Answer from the drawing. Dimensions are ordinates in mm from the lowest x, y and z of the part. A direction names the side the tool comes from. Give positions to 0.01 mm unless a question says otherwise; leave off trailing zeros. Order: outer loops, then holes, each group sorted by start corner. A loop starts at its lowest first (then second) coordinate and runs counter-clockwise, first axis right, second up. Notation, with made-up numbers: (-25, 25.25) - (34, 25.25) arc R32 ccw to (34, 62.25) - close; hole circle Ø2 at (49.25, 24.5). An arc over 180 degrees is marked (long way). One line per item, written item: value. Start each with the question number.
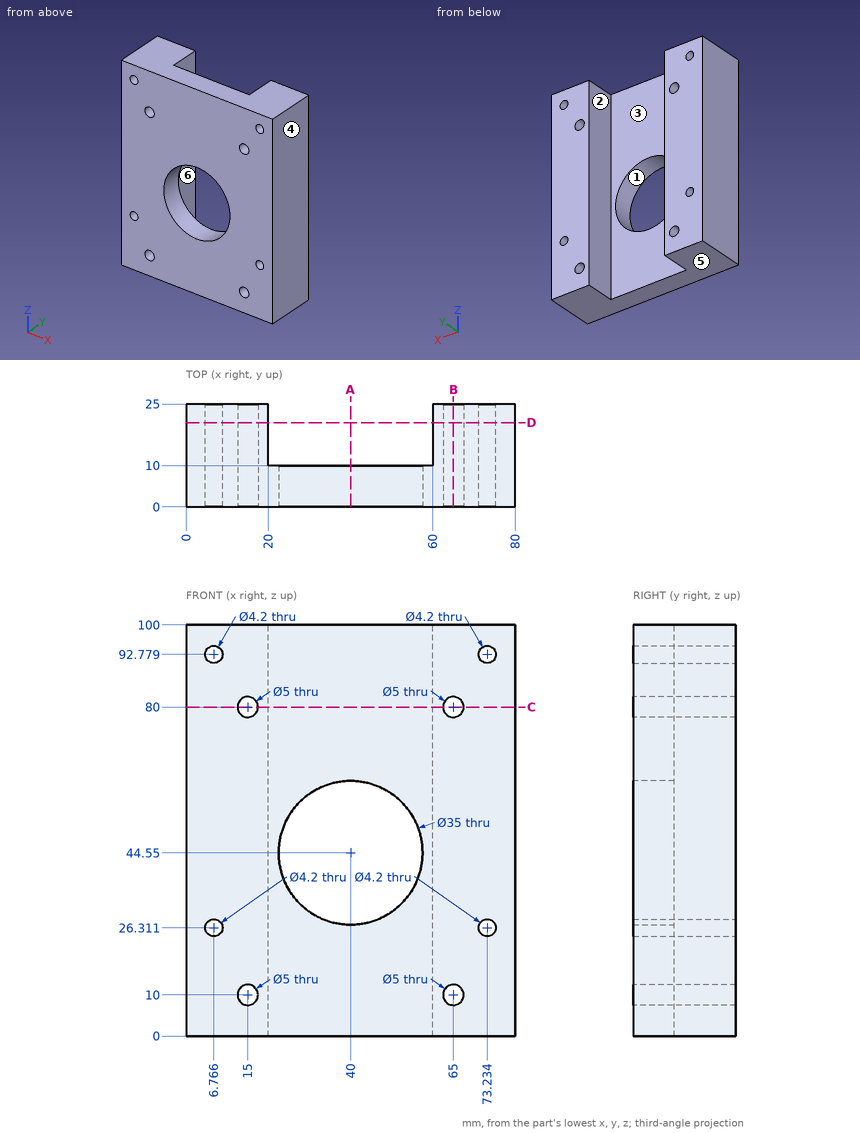
1) Section A-A on x = 40 is taken. Write down the section's boundary in (y, z).
2) This flat-tipped pin is pushed along its axis until it touches: pin 1 (3.5 mm diameter, centred on x = 6.77, z = 92.78, fed in from -Y). Where does it stop, or does it pass through?
3) Find the intervals of material crossed by probe 1 along X at (y, z) = (12.75, 11); probe 2 along X at (y, z) = (18.75, 65.5); probe 3 along X at (y, z) = (2.25, 94.5), in increasing order. Write a range as from..to.
4) Section C-C on z = 80 is taken. Write down the section's boundary in (x, y), plus the area to 3 significant figures.
5) Section B-B on x = 65 is taken. Write down the section's boundary in (y, z), plus the area to 3 significant figures.
6) The mould has two halves that part along X. Classify the marked faces 3, 4, 5 and 6: +X half, -X half, draft (parallel to the pull), parting line (faces both ways), or undercut.
7) Section D-D on y = 20.5 is taken. Give the number of separate pieces and of enclosed holes in the cut face, plus the area to 3 significant figures.
8) For the marked faces 1 and 2, determine the directions among +Z, -Z, +X, -X, +Y, -Y from which every point of the face is accessible in a straight line to the end or side of a thin tool.
Solved:
1. outline: (0, 0) - (10, 0) - (10, 27.05) - (0, 27.05) - close; (0, 62.05) - (10, 62.05) - (10, 100) - (0, 100) - close
2. pin 1: passes through
3. probe 1: x = 0..12.71, 17.29..20, 60..62.71, 67.29..80
3. probe 2: x = 0..20, 60..80
3. probe 3: x = 0..5.56, 7.97..72.03, 74.44..80
4. outline: (0, 0) - (12.5, 0) - (12.5, 25) - (0, 25) - close; (17.5, 0) - (62.5, 0) - (62.5, 25) - (60, 25) - (60, 10) - (20, 10) - (20, 25) - (17.5, 25) - close; (67.5, 0) - (80, 0) - (80, 25) - (67.5, 25) - close
4. area: 1,150 mm2
5. outline: (0, 0) - (25, 0) - (25, 7.5) - (0, 7.5) - close; (0, 12.5) - (25, 12.5) - (25, 77.5) - (0, 77.5) - close; (0, 82.5) - (25, 82.5) - (25, 100) - (0, 100) - close
5. area: 2,250 mm2
6. face 3: undercut
6. face 4: +X half
6. face 5: draft
6. face 6: undercut
7. separate pieces: 2
7. enclosed holes: 8
7. area: 3,870 mm2
8. face 1: +Y, -Y
8. face 2: +Z, -Z, +Y
